Check sheet for the modelled part. Datum: model origin and axes. Units: mm. Give positions to 0.01 mm unless a question says otherwise; leave off trailing zeros. Write each loop counter-clockwise with the first axis right and the second up, starting at its lowest first coordinate (ties: lowest second). Pieces come first, ordered by that corner, then holes. Notation, with made-up numbers: (57.5, 45.5) -> (99.5, 45.5) arc R22 cw to (99.5, 84.5) -> close; hole circle Ø11 at (-32.75, -31). An arc over 180 degrees is marked (long way). Use a Markdown table: item, result. Add a question column.
1. Cross-section at C-C (x = 2.75). Enter the section's corners in (y, z), then the cut area to 3 significant figures.
2. Release check for a two-part mould opening along X. For faces 1 (the cylindrical face through (-5.473, 0.74, 5.005)), 2 (the flat face through (3, 1, 1.573)), 3 (the flat face through (-3.84, 0.74, 0.73)) record: released by +X, released by -X, zero draft, split by the parting line, or undercut.
3. Cross-section at A-A (z = 5). Enter the section's corners in (x, y), then the cut area to 3 significant figures.
4. Gauge pin test, flat end, axial feed: P1, Ø0.8, axis at x = 2.5, y = 0.5, coming from the +Z side. Record the tip position at first contact, or that the pin passes through.
5. Scan lines: probe 1 along Z at (x, y) = (-4.25, 0.55); probe 2 along X at (y, z) = (0.4, 4.25); probe 3 along Z at (x, y) = (2.25, 0.95). Record each from-to range of solid material in increasing order. Write a range as [from, to].
6. Cross-section at B-B (y = 0.8). Enter the section's corners in (x, z), then the cut area to 3 significant figures.
7. Cross-section at D-D (z = 6.25). Enter the section's corners in (x, y).
from build123d import *

# Parameters (mm, degrees)
SKETCH_2_R      = 1.1
EXTRUDE_1_DEPTH = 1.5


with BuildPart() as part:
    # 草图2 → 凸台-拉伸1 (new body)
    with BuildSketch(Plane(origin=(0, 0, 0), x_dir=(1, 0, 0), z_dir=(0, 1, 0))):
        with BuildLine():
            Line((1.537957249, 1.537957249), (4.649227086, 1.537957249))
            Line((4.649227086, 1.537957249), (4.649227086, -1.573312588))
            Line((4.649227086, -1.573312588), (1.537957249, -1.573312588))
            Line((1.537957249, -1.573312588), (-2.94156421, -6.052834047))
            ThreePointArc((-2.94156421, -6.052834047), (-6.052834047, -6.052834047), (-6.052834047, -2.94156421))
            Line((-6.052834047, -2.94156421), (-1.573312588, 1.537957249))
            Line((-1.573312588, 1.537957249), (1.537957249, 1.537957249))
        make_face()
        with Locations(Location((-4.497199128, -4.497199128, 0), (0, 0, 270))):
            Circle(SKETCH_2_R, mode=Mode.SUBTRACT)
    extrude(amount=EXTRUDE_1_DEPTH)


solid = part.part
Worked answers:
| question | item | result |
|---|---|---|
| 1 | outline | (0, -1.54) -> (1.5, -1.54) -> (1.5, 1.57) -> (0, 1.57) -> close |
| 1 | area | 4.67 mm² |
| 2 | face 1 | undercut |
| 2 | face 2 | zero draft |
| 2 | face 3 | released by -X |
| 3 | outline | (-6.64, 0) -> (-5.48, 0) -> (-5.48, 1.5) -> (-6.64, 1.5) -> close; (-3.52, 0) -> (-1.89, 0) -> (-1.89, 1.5) -> (-3.52, 1.5) -> close |
| 3 | area | 4.19 mm² |
| 4 | P1 | stops at z = 1.57 |
| 5 | probe 1 | z = [1.14, 3.43], [5.57, 6.68] |
| 5 | probe 2 | x = [-6.68, -5.57], [-3.43, -1.14] |
| 5 | probe 3 | z = [-1.54, 1.57] |
| 6 | outline | (-6.05, 2.94) -> (-1.57, -1.54) -> (4.65, -1.54) -> (4.65, 1.57) -> (1.54, 1.57) -> (-2.94, 6.05) arc R2.2 ccw to start; hole circle Ø2.2 at (-4.5, 4.5) |
| 6 | area | 46.2 mm² |
| 7 | outline | (-5.83, 0) -> (-3.17, 0) -> (-3.17, 1.5) -> (-5.83, 1.5) -> close |
